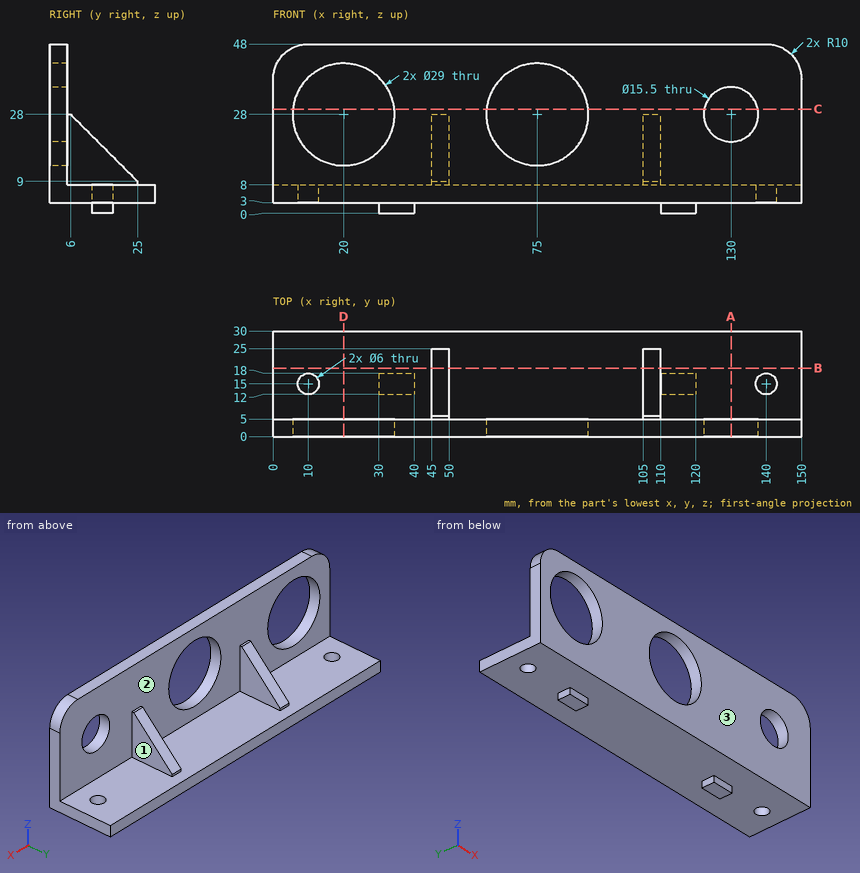
Input: dimensioned drawing with shaded views. Units: mm. Origin: part minimum x, y, z. Coordinates: 2 decimals unless noted, no trailing zeros. Loops run counter-clockwise (first coordinate to the right, second up) from the corner with the lowest first, then second, coordinate; pieces in that order, holes last. Notation, with made-up numbers: M 51,23 L 94,23 A17 ccw 94,47 Z; hole C 6,11 d9. An arc over 180 degrees is marked long. Use a Markdown table: item, result. Add a question column.
Q1. Section query D-D, the plane x = 20. Return loops of the section in (y, z), and give its area (3 significant figures).
Q2. Section query C-C, the plane z = 29.5. Return loops of the section in (x, y).
Q3. Section query A-A, the plane x = 130. Return loops of the section in (y, z).
Q4. First-contact query: pin 1 (6 mm diameter, centred on y = 17.5, z = 17.5, fed in from -X); pin 2 (0.8 mm diameter, centred on x = 48.5, y = 5.5, fed in from +Z); pin 3 (1.5 mm diameter, centred on y = 16, z = 1.5, fed in from -X); pin 4 (3.5 mm diameter, centred on x = 33.5, z = 2, fed in from -Y). Flat tips, straight axial feed; report the tip coordinate or a pass-through.
Q5. Draft query along X for the marked faces 1, 2 and 3. Return one class per face: pulls with the +X half, pulls with the -X half, needs draft (parallel to the pull), parting line crosses it, or undercut.
Q6. Material intervals for L1, parallel to X at y = 15, z = 6.35; L2, parallel to Z at x = 20, y = 2.1; L3, parallel to X at y = 16.25, z = 8.5, sorted ascending.
Q7. Section query B-B, the plane y = 19.5. Return loops of the section in (x, z), and give its area (3 significant figures).
Result:
| question | item | result |
|---|---|---|
| 1 | outline | M 0,3 L 30,3 L 30,8 L 5,8 L 5,13.5 L 0,13.5 Z; M 0,42.5 L 5,42.5 L 5,48 L 0,48 Z |
| 1 | area | 205 mm2 |
| 2 | outline | M 0,0 L 5.58,0 L 5.58,5 L 0,5 Z; M 34.42,0 L 60.58,0 L 60.58,5 L 34.42,5 Z; M 89.42,0 L 122.4,0 L 122.4,5 L 89.42,5 Z; M 137.6,0 L 150,0 L 150,5 L 137.6,5 Z |
| 3 | outline | M 0,3 L 30,3 L 30,8 L 5,8 L 5,20.25 L 0,20.25 Z; M 0,35.75 L 5,35.75 L 5,48 L 0,48 Z |
| 4 | pin 1 | stops at x = 45 |
| 4 | pin 2 | stops at z = 28 |
| 4 | pin 3 | stops at x = 30 |
| 4 | pin 4 | stops at y = 0 |
| 5 | face 1 | pulls with the +X half |
| 5 | face 2 | undercut |
| 5 | face 3 | needs draft |
| 6 | L1 | x = 0 to 7, 13 to 137, 143 to 150 |
| 6 | L2 | z = 3 to 13.5, 42.5 to 48 |
| 6 | L3 | x = 45 to 50, 105 to 110 |
| 7 | outline | M 0,3 L 150,3 L 150,8 L 110,8 L 110,14.5 L 105,14.5 L 105,8 L 50,8 L 50,14.5 L 45,14.5 L 45,8 L 0,8 Z |
| 7 | area | 815 mm2 |
